Work out the finished part from the listing and answer in its coordinate system (mm). A direction names the side the tool comes from. Round coordinates to 2 decimals unless told otherwise and drop trailing zeros. Write each loop counter-clockwise with the first axis right and the second up, starting at its lowest first coordinate (ties: lowest second). Pieces come first, ordered by that corner, then holes. Notation, with made-up numbers: M -5.5,88.25 L 14.5,88.25 A17 cw 14.5,113.25 Z; hole C 6.5,38 d7. An arc over 180 degrees is marked long. One line per item, written item: value. Start each with the question number.
Q1. Find section C-C (z = 39). Write down the section's boundary in (x, y), and give its area (3 significant figures).
Q2. Consider probe 1 along X at (y, z) = (1.5, 38.5); probe 2 along X at (y, z) = (47.5, 28); probe 3 along Y at (x, z) = (11, 26.5). Determine where each line is inside the solid, lowest interval first.
Q3. Given pin 1 Ø6 at (x, z) = (3, 25) entering from +Y; pin 2 Ø6 at (x, z) = (5.5, 30.5) entering from -Y; pin 3 Ø1.5 at (x, y) = (17, 16) entering from +Z (3 decimals), each flat-ended and moving along its own axis, determine where each tip first touches the part or whether it passes through.
Q4. A tool of negligible diameter and unlimited length cuts with its end or side. For faces 1 (the cylindrical face through (-37.59, -23.96, 2.03)), 2 (the flat face through (-7, 1, 9.525)), 3 (the flat face through (-6, 1, 0)), from which of +Z, -Z, +X, -X, +Y, -Y can it reach the whole face along a straight path? Write none if from no direction.
Q5. Find section D-D (z = 30). Write down the section's boundary in (x, y).
from build123d import *


with BuildPart() as f1:
    # F0 (on Front) → F1 (revolve)
    with BuildSketch(Plane.XZ):
        with BuildLine():
            ThreePointArc((62.848027, 43.741147), (62.637688, 45.096197), (61.416511, 45.72))
            Line((61.416511, 45.72), (61.416267, 45.72))
            ThreePointArc((61.416267, 45.72), (60.532359, 45.433605), (59.984365, 44.68326))
            Line((59.984365, 44.68326), (53.599079, 25.249327))
            ThreePointArc((53.599079, 25.249327), (45.28761, 13.868776), (31.881304, 9.525))
            Line((31.881304, 9.525), (25.4, 9.525))
            Line((25.4, 9.525), (0, 9.525))
            Line((0, 9.525), (-6.35, 9.525))
            Line((-6.35, 9.525), (-6.35, 0))
            Line((-6.35, 0), (0, 0))
            Line((0, 0), (24.376065, 0))
            Line((24.376065, 0), (31.321423, 0))
            Line((31.321423, 0), (33.02, 0))
            Line((33.02, 0), (33.02, 3.996068))
            ThreePointArc((33.02, 3.996068), (33.657398, 5.678835), (35.249688, 6.517042))
            ThreePointArc((35.249688, 6.517042), (48.265616, 12.09679), (56.270939, 23.778518))
            Line((56.270939, 23.778518), (62.848027, 43.741147))
        make_face()
    revolve(axis=Axis((-6.35, 0, 4.7625), (0, 0, 1)))


solid = f1.part
The answers:
1. outline: C -6.35,0 d135.27; hole C -6.35,0 d128.93
1. area: 1,320 mm2
2. probe 1: -73.8 to -70.64, 57.94 to 61.1
2. probe 2: -49.26 to -44.39, 31.69 to 36.56
2. probe 3: -61.1 to -57.81, 57.81 to 61.1
3. pin 1: y = 63.41
3. pin 2: y = -64.87
3. pin 3: z = 9.525
4. face 1: -Z
4. face 2: +Z
4. face 3: -Z, +X, -X, +Y, -Y
5. outline: C -6.35,0 d129.34; hole C -6.35,0 d123.02
